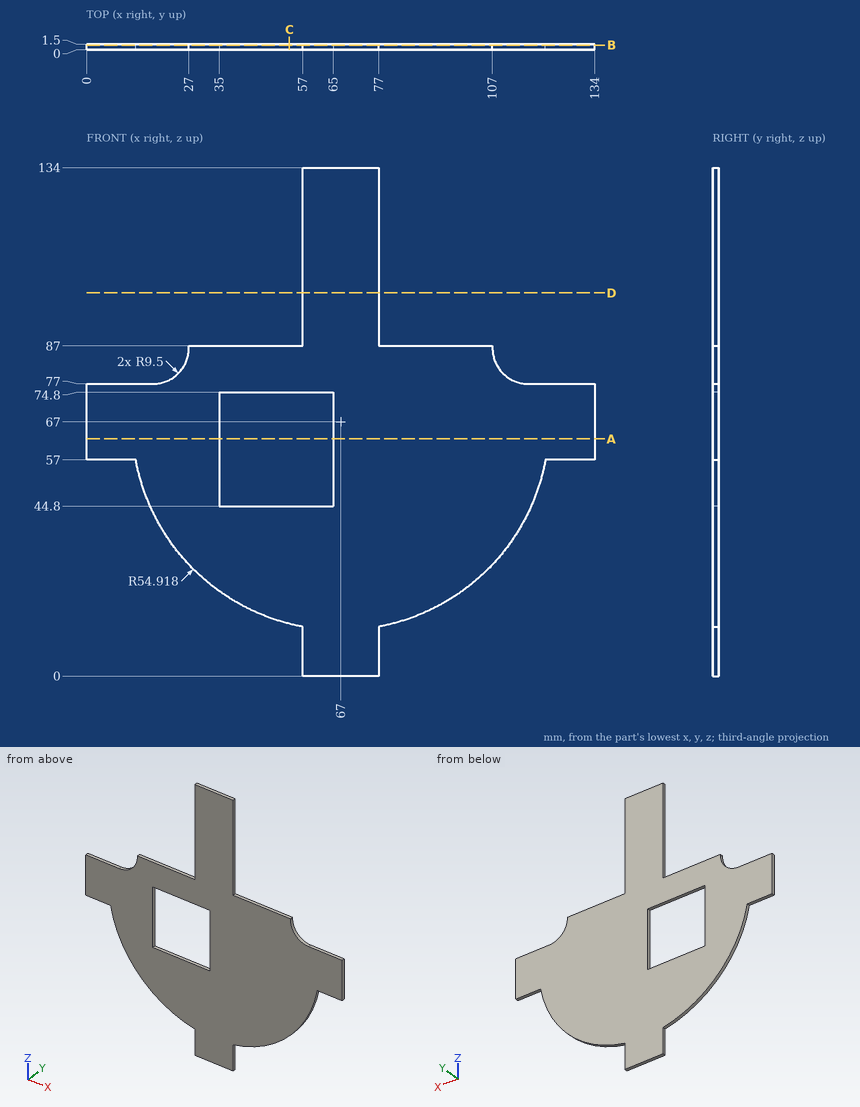
Check sheet for the drawn part. Datum: minimum x, y, z corner. Units: mm. Round coordinates to 2 decimals unless told otherwise and drop trailing zeros. Order: outer loops, then holes, each group sorted by start corner. A loop starts at its lowest first (then second) coordinate and runs counter-clockwise, first axis right, second up. Notation, with made-up numbers: (72.5, 56.25) -> (128.5, 56.25) arc R23 ccw to (128.5, 74.25) -> close; hole circle Ø7 at (68, -25.75). An arc over 180 degrees is marked (long way). Put each result on its own line as item: value. Start each with the question number.
(1) Section check D-D (z = 101). Enter the section's corners in (x, y), then the cut area to 3 significant figures.
(2) Depth check by flat-ended pin: pin 1 Ø0.8 at (x, y) = (127, 0.5) entering from -Z; pin 2 Ø0.6 at (y, z) = (0.5, 86.5) entering from +X; pin 3 Ø0.8 at (x, y) = (52, 1) entering from -Z. Enter the tip coordinate at first touch or a pass-through.
(3) Section check C-C (x = 53.5). Enter the section's corners in (y, z).
(4) Material ranges on line 1 along X through (y, z) = (0.95, 70); line 2 along X through (y, z) = (1.25, 103); line 3 along Z through (x, y) = (44.5, 0.1), recorded low to high.
(5) Section check A-A (z = 62.5). Enter the section's corners in (x, y), then the cut area to 3 significant figures.
(6) Section check B-B (y = 1.2). Enter the section's corners in (x, z).
Completed:
1. outline: (57, 0) -> (77, 0) -> (77, 1.5) -> (57, 1.5) -> close
1. area: 30.0 mm2
2. pin 1: stops at z = 57
2. pin 2: stops at x = 107
2. pin 3: stops at z = 14.06
3. outline: (0, 13.77) -> (1.5, 13.77) -> (1.5, 44.8) -> (0, 44.8) -> close; (0, 74.8) -> (1.5, 74.8) -> (1.5, 87) -> (0, 87) -> close
4. line 1: x = 0 to 35, 65 to 134
4. line 2: x = 57 to 77
4. line 3: z = 16.9 to 44.8, 74.8 to 87
5. outline: (0, 0) -> (35, 0) -> (35, 1.5) -> (0, 1.5) -> close; (65, 0) -> (134, 0) -> (134, 1.5) -> (65, 1.5) -> close
5. area: 156 mm2
6. outline: (0, 57) -> (13, 57) arc R54.92 ccw to (57, 13) -> (57, 0) -> (77, 0) -> (77, 13) arc R54.92 ccw to (121, 57) -> (134, 57) -> (134, 77) -> (116.5, 77) arc R9.5 cw to (107, 86.5) -> (107, 87) -> (77, 87) -> (77, 134) -> (57, 134) -> (57, 87) -> (27, 87) -> (27, 86.5) arc R9.5 cw to (17.5, 77) -> (0, 77) -> close; hole (35, 44.8) -> (65, 44.8) -> (65, 74.8) -> (35, 74.8) -> close
